For this review, use the dimensioned drawing (mm, ordinates from the lowest corner) and the shaded views. Round coordinates to 2 decimals unless told otherwise and drop trailing zeros. Order: outer loops, then holes, each group sorted by start corner. A loop starts at its lowest first (then second) coordinate and runs counter-clockwise, first axis right, second up. Notation, with made-up numbers: (-16, -30) -> (25, -30) arc R13 cw to (25, -25) -> close; hole circle Ø1 at (-20.75, -28.75). An arc over 180 degrees is marked (long way). Answer in a Markdown table with one row per item.
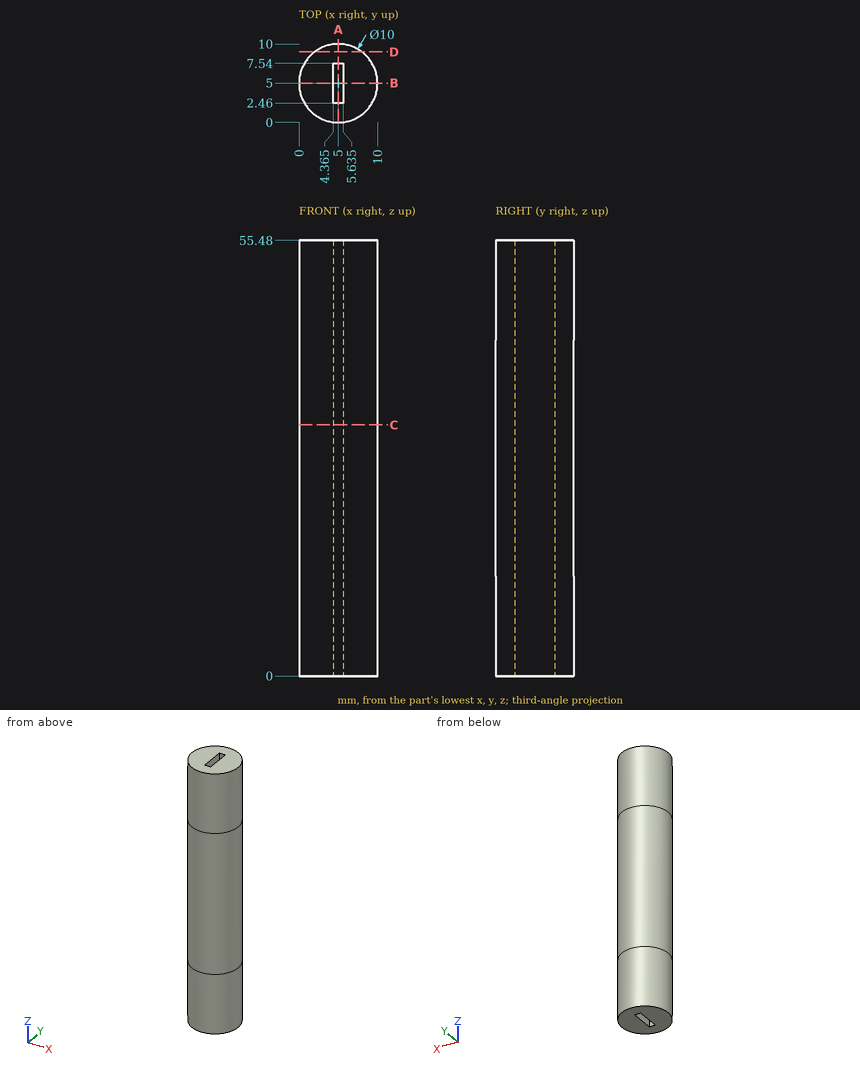
Q1. Take a section at A-A, the plane x = 5. Write out the cut boundary in (y, z), then the cut area to 3 significant figures.
Answer key:
| item | result |
|---|---|
| outline | (0, 0) -> (2.46, 0) -> (2.46, 55.48) -> (0, 55.48) -> close; (7.54, 0) -> (10, 0) -> (10, 55.48) -> (7.54, 55.48) -> close |
| area | 273 mm^2 |
Q2. Take a section at D-D, the plane y = 9. Write out the cut boundary in (x, z).
Answer key:
| item | result |
|---|---|
| outline | (2, 0) -> (8, 0) -> (8, 55.48) -> (2, 55.48) -> close |
Q3. Clearance check with flat-ended pins moving along their axes: pin 1 Ø2 at (y, z) = (1.5, 38.5) entering from +X; pin 2 Ø1 at (y, z) = (3, 35.5) entering from +X; pin 3 Ø6 at (x, z) = (6, 32) entering from -Y. State where each tip first meets the part, or that it passes through.
Answer key:
| item | result |
|---|---|
| pin 1 | stops at x = 9.33 |
| pin 2 | stops at x = 9.77 |
| pin 3 | stops at y = 0 |
Q4. To check wall thickness, follow probe 1 along X at (y, z) = (5.25, 28.5) (3 decimals); probe 2 along Y at (x, z) = (5.25, 50); probe 3 along X at (y, z) = (5.75, 40.5) (3 decimals). State the ranges of each line that lie inside material, in increasing order.
Answer key:
| item | result |
|---|---|
| probe 1 | x = 0.006 to 4.365, 5.635 to 9.994 |
| probe 2 | y = 0.01 to 2.46, 7.54 to 9.99 |
| probe 3 | x = 0.057 to 4.365, 5.635 to 9.943 |
Q5. Take a section at B-B, the plane y = 5. Write out the cut boundary in (x, z) (3 decimals), then the cut area to 3 significant figures.
Answer key:
| item | result |
|---|---|
| outline | (0, 0) -> (4.365, 0) -> (4.365, 55.48) -> (0, 55.48) -> close; (5.635, 0) -> (10, 0) -> (10, 55.48) -> (5.635, 55.48) -> close |
| area | 484 mm^2 |
Q6. Take a section at C-C, the plane z = 32. Write out the cut boundary in (x, y) (3 decimals).
Answer key:
| item | result |
|---|---|
| outline | circle Ø10 at (5, 5); hole (4.365, 2.46) -> (5.635, 2.46) -> (5.635, 7.54) -> (4.365, 7.54) -> close |
